```python
from build123d import *

# Parameters (mm, degrees)
SKETCH_1_R          = 13.95
EXTRUDE_1_DEPTH     = 12.8
CUT_EXTRUDE_1_DEPTH = 20


with BuildPart() as part:
    # 草图1 → 凸台-拉伸1 (new body)
    with BuildSketch(Plane(origin=(0, 0, 0), x_dir=(1, 0, 0), z_dir=(0, 1, 0))):
        with Locations(Location((0, 0, 0), (0, 0, 270))):
            Circle(SKETCH_1_R)
    extrude(amount=EXTRUDE_1_DEPTH)

    # 草图2 → 切除-拉伸1 (cut)
    with BuildSketch(Plane(origin=(0, 12.8, 0), x_dir=(1, 0, 0), z_dir=(0, 1, 0))):
        with BuildLine():
            Line((2.4, 1), (3.2, 1))
            Line((3.2, 1), (3.2, -1))
            Line((3.2, -1), (2.4, -1))
            ThreePointArc((2.4, -1), (-2.6, 0), (2.4, 1))
        make_face()
    extrude(amount=-CUT_EXTRUDE_1_DEPTH, mode=Mode.SUBTRACT)

    # 草图6 → 旋转1 (revolve)
    with BuildSketch(Plane.XY, mode=Mode.PRIVATE) as revolve_1_sk:
        Polygon((12.14125, 12.3), (12.14125, 12.8), (13.95, 12.8), (15.871025404, 13.314737206), (16.005, 12.814737206), (14.083974596, 12.3), align=None)
    revolve(revolve_1_sk.sketch.rotate(Axis((0, 0, 0), (0, 1, 0)), 90), axis=Axis((0, 0, 0), (0, 1, 0)))

    # 草图8 → 旋转2 (revolve)
    with BuildSketch(Plane.XY):
        Polygon((12.14125, 0.5), (12.14125, 0), (13.95, 0), (15.871025404, -0.514737206), (16.005, -0.014737206), (14.083974596, 0.5), align=None)
    revolve(axis=Axis((0, 0, 0), (0, 1, 0)))


solid = part.part
```
Geometry: final body of the model. Coordinates: model frame, mm. A direction names the side the tool comes from. Coordinates: 2 decimals unless noted, no trailing zeros. Order: outer loops, then holes, each group sorted by start corner. A loop starts at its lowest first (then second) coordinate and runs counter-clockwise, first axis right, second up. Notation, with made-up numbers: (77, -8.5) - (111, -8.5) arc R31 ccw to (111, 16.5) - close; hole circle Ø8 at (9, 26). An arc over 180 degrees is marked (long way). Write each question's results on one line, items separated by ' | '.
1) Set-up query: faces 1 (the flat face through (3.2, 6, 0)), 2 (the flat face through (-3, 12.8, 0)). Return all of +Z, -Z, +X, -X, +Y, -Y with unobstructed straight access to the full face (end or side cutting, diameter ignored); none if empty.
Results list:
face 1: +Y, -Y | face 2: +Y
2) Line query: line 1 (Z direction, x = 0, y = 6); line 2 (X direction, y = 4.25, z = 0); line 3 (Y direction, x = 1.5, z = -4.5). Output: solid intervals per line, ascending. Write a range as from..to.
Results list:
line 1: -13.95..-2.6, 2.6..13.95 | line 2: -13.95..-2.6, 3.2..13.95 | line 3: 0..12.8
3) Section A-A, the plane z = 0. Return loops of the section in (x, y) (3 decimals).
Results list:
outline: (-16.005, -0.015) - (-15.871, -0.515) - (-13.95, 0) - (-2.6, 0) - (-2.6, 12.8) - (-13.95, 12.8) - (-15.871, 13.315) - (-16.005, 12.815) - (-14.084, 12.3) - (-13.95, 12.3) - (-13.95, 0.5) - (-14.084, 0.5) - close; (3.2, 0) - (13.95, 0) - (15.871, -0.515) - (16.005, -0.015) - (14.084, 0.5) - (13.95, 0.5) - (13.95, 12.3) - (14.084, 12.3) - (16.005, 12.815) - (15.871, 13.315) - (13.95, 12.8) - (3.2, 12.8) - close
4) Section C-C, the plane y = 10.5. Return loops of the section in (x, z).
Results list:
outline: circle Ø27.9 at (0, 0); hole (2.4, -1) - (3.2, -1) - (3.2, 1) - (2.4, 1) arc R2.6 ccw (long way) to start
5) Pull-direction query (Y, two-part tool) for faces 3 (the cylindrical face through (-13.62, 6.32, -3.02)), 4 (the flat face through (3, 6, 1)), 5 (the flat face through (-3, 0, 0)); classes: pulls with the +Y half, pulls with the -Y half, needs draft (parallel to the pull), parting line crosses it, or undercut.
Results list:
face 3: undercut | face 4: needs draft | face 5: pulls with the -Y half
6) Section B-B, the plane x = 0. Return loops of the section in (y, z) (3 decimals).
Results list:
outline: (-0.515, -15.871) - (-0.015, -16.005) - (0.5, -14.084) - (0.5, -13.95) - (12.3, -13.95) - (12.3, -14.084) - (12.815, -16.005) - (13.315, -15.871) - (12.8, -13.95) - (12.8, -2.6) - (0, -2.6) - (0, -13.95) - close; (-0.515, 15.871) - (0, 13.95) - (0, 2.6) - (12.8, 2.6) - (12.8, 13.95) - (13.315, 15.871) - (12.815, 16.005) - (12.3, 14.084) - (12.3, 13.95) - (0.5, 13.95) - (0.5, 14.084) - (-0.015, 16.005) - close
7) Pin query (flat end, axial travel): pin 1 (1.5 mm diameter, centred on x = -9, y = 5.5, fed in from -Z); pin 2 (8.5 mm diameter, centred on x = -6.5, z = 3, fed in from +Y); pin 3 (0.9 mm diameter, centred on x = 3, y = 8, fed in from -Z). Return the tip coordinate at first contact, or that it passes through.
Results list:
pin 1: z = -11.25 | pin 2: y = 12.8 | pin 3: z = -13.71
